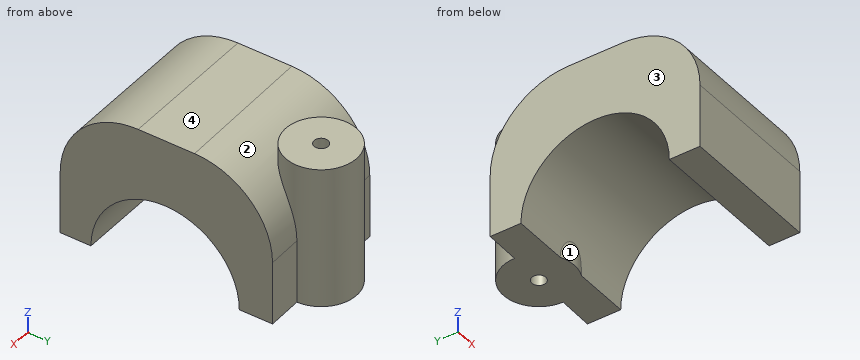
from build123d import *

# Parameters (mm, degrees)
F1_DEPTH  = 7.493
F3_DEPTH  = 10.0086
F5_DEPTH  = 2.4892
F6_R      = 5.5118
F7_R      = 2.5019
F8_DEPTH  = 9.9822
F9_R      = 0.4953
F10_DEPTH = 9.9822


with BuildPart() as f1:
    # F0 (on Top) → F1 (new body)
    with BuildSketch(Plane.XY):
        Polygon((-14.141997, 3.073401), (-14.141997, -11.759634), (-4.134397, -11.759634), (-4.134397, 3.251766), align=None)
    extrude(amount=F1_DEPTH)

    # F2 (on face) → F3 (cut, through all)
    with BuildSketch(Plane(origin=(-14.141997, 0, 0), x_dir=(0, -1, 0), z_dir=(-1, 0, 0))):
        with BuildLine():
            Line((-0.901983, 0), (9.588217, 0))
            ThreePointArc((9.588217, 0), (4.343117, 5.2451), (-0.901983, 0))
        make_face()
    extrude(amount=-F3_DEPTH, mode=Mode.SUBTRACT)

    # F4 (on face) → F5 (join)
    with BuildSketch(Plane.XY.offset(7.493)):
        Polygon((-4.134397, 3.251766), (-14.141997, 3.073401), (-14.141997, -11.759634), (-4.134397, -11.759634), align=None)
    extrude(amount=F5_DEPTH)

    # F6
    f6_edges = [f1.edges().sort_by_distance(p)[0] for p in [
        (-9.138197, 3.162583, 9.9822),
        (-9.138197, -11.759634, 9.9822),
    ]]
    fillet(f6_edges, radius=F6_R)

    # F7 (on face) → F8 (join)
    with BuildSketch(Plane.XY.offset(9.9822)):
        with Locations((-9.138197, 3.162583)):
            Circle(F7_R)
    extrude(amount=-F8_DEPTH)

    # F9 (on face) → F10 (cut)
    with BuildSketch(Plane.XY.offset(9.9822)):
        with Locations((-9.138197, 3.162583)):
            Circle(F9_R)
    extrude(amount=-F10_DEPTH, mode=Mode.SUBTRACT)


solid = f1.part
Input: part model. Units: mm. Frame: model coordinates. Face numbers are marked on the shaded views. Round coordinates to 2 decimals unless told otherwise and drop trailing zeros. Write each loop counter-clockwise with the first axis right and the second up, starting at its lowest first coordinate (ties: lowest second). Pieces come first, ordered by that corner, then holes.
1) Ray query, L1, parallel to Y at x = -10.25, z = 4.5; L2, parallel to X at y = 3.5, z = 0.75; L3, parallel to Y at x = -11.75, z = 1. Return the intervals inside material, ascending.
2) Cut plane D-D (y = -9.25). Return the cut outline in (x, z), then the cut area to 3 significant figures.
3) Cut plane A-A (z = 3). Return the cut outline in (x, y), then the cut area to 3 significant figures.
4) Cut plane B-B (z = 8.5). Return the cut outline in (x, y), then the cut area to 3 significant figures.
5) Cut plane C-C (y = -7.5). Return the cut outline in (x, z), then the cut area to 3 significant figures.
6) Draft query along X for the marked faces 1, 2, 3 and 4. Return one class per face: pulls with the +X half, pulls with the -X half, needs draft (parallel to the pull), parting line crosses it, or undercut.
7) Contact query for flat-ended pins moving along their axis: P1, Ø1.5, axis at x = -8.5, y = -9.5, coming from the +Z side; P2, Ø5, axis at x = -5.5, z = 4, coming from the +Y side; P3, Ø4, axis at x = -5, z = 7, coming from the -Y side. Output: stop coordinate, or through.
Geometry says:
1. L1: y = -11.76 to -7.04, -1.65 to 5.4
1. L2: x = -11.62 to -9.5, -8.78 to -6.66
1. L3: y = -11.76 to -9.49, 0.81 to 3.12
2. outline: (-14.14, 1.85) - (-4.13, 1.85) - (-4.13, 9.09) - (-14.14, 9.09) - close
2. area: 72.5 mm2
3. outline: (-14.14, -11.76) - (-4.13, -11.76) - (-4.13, -8.65) - (-14.14, -8.65) - close; (-14.14, -0.04) - (-4.13, -0.04) - (-4.13, 3.25) - (-6.64, 3.21) arc R2.5 ccw to (-11.64, 3.12) - (-14.14, 3.07) - close; hole circle Ø0.99 at (-9.14, 3.16)
3. area: 72.3 mm2
4. outline: (-14.14, -10.01) - (-4.13, -10.01) - (-4.13, 1.5) - (-7.32, 1.44) arc R2.5 ccw (long way) to (-10.89, 1.38) - (-14.14, 1.32) - close; hole circle Ø0.99 at (-9.14, 3.16)
4. area: 131 mm2
5. outline: (-14.14, 4.19) - (-4.13, 4.19) - (-4.13, 9.84) - (-14.14, 9.84) - close
5. area: 56.5 mm2
6. face 1: parting line crosses it
6. face 2: undercut
6. face 3: pulls with the -X half
6. face 4: needs draft
7. P1: stops at z = 9.38
7. P2: stops at y = 5.39
7. P3: stops at y = -11.73
